The listing builds one solid part. Answer for the finished solid, in the listing's coordinates (mm). A direction names the side the tool comes from. Coordinates: 2 decimals unless noted, no trailing zeros. Order: outer loops, then holes, each group sorted by start corner. A loop starts at its lowest first (then second) coordinate and runs counter-clockwise, first axis right, second up. Notation, with made-up numbers: (-29, -26) -> (-4, -26) arc R22 ccw to (-4, 10) -> close; hole circle Ø7 at (1.25, 87.5). An arc over 180 degrees is marked (long way). Answer in a Markdown table with one row per item.
```python
from build123d import *

# Parameters (mm, degrees)
F0_W     = 60
F0_H     = 40
F1_DEPTH = 10
F4_DEPTH = 40
F5_DEPTH = 25
F7_DEPTH = 40


with BuildPart() as f1:
    # F0 (on Top) → F1 (new body)
    with BuildSketch(Plane.XY):
        Rectangle(F0_W, F0_H)
    extrude(amount=F1_DEPTH)

    # F3 (on face) → F4 (join)
    with BuildSketch(Plane.XZ.offset(20)):
        Polygon((0, 0), (14.609862, 10), (-30, 10), (-30, 0), align=None)
    extrude(amount=-F4_DEPTH)

    # F2 (on face) → F5 (cut)
    with BuildSketch(Plane.XY.offset(10)):
        with BuildLine():
            ThreePointArc((0, 11.150862), (2.75, 13.900862), (0, 16.650862))
            Line((0, 16.650862), (-23.533953, 16.650862))
            ThreePointArc((-23.533953, 16.650862), (-26.283953, 13.900862), (-23.533953, 11.150862))
            Line((-23.533953, 11.150862), (0, 11.150862))
        make_face()
        with BuildLine():
            ThreePointArc((0, -13.849138), (2.75, -11.099138), (0, -8.349138))
            Line((0, -8.349138), (-23.533953, -8.349138))
            ThreePointArc((-23.533953, -8.349138), (-26.283953, -11.099138), (-23.533953, -13.849138))
            Line((-23.533953, -13.849138), (0, -13.849138))
        make_face()
    extrude(amount=-F5_DEPTH, mode=Mode.SUBTRACT)

    # F6 (on face) → F7 (cut)
    with BuildSketch(Plane.XZ.offset(20)):
        Polygon((30, 0), (30, 10), (14.609862, 0), align=None)
    extrude(amount=-F7_DEPTH, mode=Mode.SUBTRACT)


solid = f1.part
```
(1) For a pull along X with two mould halves and no side action, classify faces 1 (the flat face through (-7, 20, 5)), 2 (the flat face through (-30, 0, 5)), 3 (the cylindrical face through (2.75, 13.84, 5.07)) as released by +X, released by -X, zero draft, split by the parting line, or undercut.
Check values:
| item | result |
|---|---|
| face 1 | zero draft |
| face 2 | released by -X |
| face 3 | undercut |
(2) Find the intervals of material crossed by line 1 along Y through (x, z) = (-23.5, 6); line 2 along Y through (x, z) = (2, 1); line 3 along X through (y, z) = (-12, 7.25), in increasing order. Write a range as from..to.
Check values:
| item | result |
|---|---|
| line 1 | -20..-13.85, -8.35..11.15, 16.65..20 |
| line 2 | -20..-12.99, -9.21..12.01, 15.79..20 |
| line 3 | -30..-26.13, 2.6..25.77 |
(3) Which of the six approach directions +Z, -Z, +X, -X, +Y, -Y give full straight-line access (tool end or side, diameter ignored) to faces 4 (the flat face through (0, 0, 10)), 5 (the cylindrical face through (-26.283, -11.039, 5.07))?
Check values:
| item | result |
|---|---|
| face 4 | +Z, +X, -X, +Y, -Y |
| face 5 | +Z, -Z |
(4) A cutting plane is placed at A-A, the plane x = -6.5. Determine the outline of the cut face in (y, z).
Check values:
| item | result |
|---|---|
| outline | (-20, 0) -> (-13.85, 0) -> (-13.85, 10) -> (-20, 10) -> close; (-8.35, 0) -> (11.15, 0) -> (11.15, 10) -> (-8.35, 10) -> close; (16.65, 0) -> (20, 0) -> (20, 10) -> (16.65, 10) -> close |
(5) A cutting plane is placed at D-D, the plane y = -2. Determine the outline of the cut face in (x, z).
Check values:
| item | result |
|---|---|
| outline | (-30, 0) -> (14.61, 0) -> (30, 10) -> (-30, 10) -> close |
(6) A cutting plane is placed at C-C, the plane x = 1. Determine the outline of the cut face in (y, z).
Check values:
| item | result |
|---|---|
| outline | (-20, 0) -> (-13.66, 0) -> (-13.66, 10) -> (-20, 10) -> close; (-8.54, 0) -> (11.34, 0) -> (11.34, 10) -> (-8.54, 10) -> close; (16.46, 0) -> (20, 0) -> (20, 10) -> (16.46, 10) -> close |
(7) A cutting plane is placed at B-B, the plane z = 6.25. Determine the outline of the cut face in (x, y).
Check values:
| item | result |
|---|---|
| outline | (-30, -20) -> (24.23, -20) -> (24.23, 20) -> (-30, 20) -> close; hole (-23.53, -13.85) -> (0, -13.85) arc R2.75 ccw to (0, -8.35) -> (-23.53, -8.35) arc R2.75 ccw to start; hole (-23.53, 11.15) -> (0, 11.15) arc R2.75 ccw to (0, 16.65) -> (-23.53, 16.65) arc R2.75 ccw to start |
(8) Flat-ended cylindrical pins translate along their axes: pin 1 (1.5 mm diameter, centred on x = 17.5, y = -5, fed in from -Z); pin 2 (2 mm diameter, centred on y = -7.5, z = 3.5, fed in from +X); pin 3 (2 mm diameter, centred on x = -8, y = -11, fed in from +Z). Find the tip coordinate at first contact, or state that the pin passes through.
Check values:
| item | result |
|---|---|
| pin 1 | z = 1.39 |
| pin 2 | x = 21.54 |
| pin 3 | through |
